Here's how the part is built. I have some questions about the finished solid (model axes, mm). A direction names the side the tool comes from. Coordinates: 2 decimals unless noted, no trailing zeros. Loops run counter-clockwise (first coordinate to the right, second up) from the corner with the lowest first, then second, coordinate; pieces in that order, holes last. Notation, with made-up numbers: M 59.25,27.25 L 84.25,27.25 A17 ccw 84.25,43.25 Z; hole C 38.25,-6.5 d6. An arc over 180 degrees is marked long. Use CSV: the item, a comma, the result in double quotes. Start each with the question number.
Q1. If we section it at C-C (y = -1.5): Please give me the cut outline in (x, z).
Q2. If we section it at B-B (x = 10.75): Please give me the cut outline in (y, z), and give its area (3 significant figures).
Q3. Please list where these lines run through material, in increasing order: probe 1 along X at (y, z) = (-7.5, 2.9); probe 2 along Y at (x, z) = (18.25, 2.5); probe 3 along Y at (x, z) = (4.5, 5). Write a range as [from, to].
Q4. For pin 1 Ø3 at (x, z) = (14, 2.5) entering from -Y; pin 2 Ø1.5 at (y, z) = (-10.5, 3) entering from +X, each with a flat end and sliding along its axis, tell me the tip position at first contact or that it passes through.
Q5. Which directions (+Z, -Z, +X, -X, +Y, -Y) give clear straight access to the entire face, cutting with the end or side of a thin tool? Please do faces 1 (the flat face through (17, 6.07, 3)), 2 (the flat face through (17, 7.45, 3)).
Q6. If we section it at A-A (z = 2.2): Please give me the cut outline in (x, y).
from build123d import *

# Parameters (mm, degrees)
SKETCH001_W = 1.38
SKETCH001_H = 6


with BuildPart() as part:
    # AdditivePipe: sweep along a path in Sketch002
    with BuildLine(Plane.XY) as additivepipe_path:
        Line((27.45, 6.07), (7.45, 6.07))
        ThreePointArc((7.45, 6.07), (3.157862, 4.292138), (1.38, 0))
        Line((1.38, 0), (1.38, -20))
    # Sketch001 → AdditivePipe (sweep)
    with BuildSketch(Plane.XZ):
        with Locations((0.69, 3)):
            Rectangle(SKETCH001_W, SKETCH001_H)
    sweep(path=additivepipe_path.line)


solid = part.part
Results below:
1,outline,"M 0,0 L 1.38,0 L 1.38,6 L 0,6 Z"
2,outline,"M 6.07,0 L 7.45,0 L 7.45,6 L 6.07,6 Z"
2,area,"8.28 mm^2"
3,probe 1,"[0, 1.38]"
3,probe 2,"[6.07, 7.45]"
3,probe 3,"[5.3, 6.84]"
4,pin 1,"y = 6.07"
4,pin 2,"x = 1.38"
5,face 1,"+Z, -Z, +X, -Y"
5,face 2,"+Z, -Z, +X, -X, +Y"
6,outline,"M 0,-20 L 1.38,-20 L 1.38,0 A6.07 cw 7.45,6.07 L 27.45,6.07 L 27.45,7.45 L 7.45,7.45 A7.45 ccw 0,0 Z"
